```python
from build123d import *

# Parameters (mm, degrees)
SKETCH1_R           = 141.81
SKETCH1_R_2         = 119.99
BOSS_EXTRUDE1_DEPTH = 10.91
CUT_EXTRUDE1_START  = -10.91
SKETCH2_W           = 21.82
SKETCH2_H           = 10.91
SKETCH2_W_2         = 10.91
SKETCH2_H_2         = 21.82
CUT_EXTRUDE1_DEPTH  = 10.91
SKETCH3_R           = 5.455
CUT_EXTRUDE2_DEPTH  = 10.91


with BuildPart() as part:
    # Sketch1 → Boss-Extrude1 (new body)
    with BuildSketch(Plane(origin=(0, 0, 0), x_dir=(1, 0, 0), z_dir=(0, 1, 0))):
        with Locations(Location((0, 0, 0), (0, 0, 270))):
            Circle(SKETCH1_R)
        with Locations(Location((0, 0, 0), (0, 0, 270))):
            Circle(SKETCH1_R_2, mode=Mode.SUBTRACT)
    extrude(amount=BOSS_EXTRUDE1_DEPTH)

    # Sketch2 → Cut-Extrude1 (cut)
    with BuildSketch(Plane(origin=(0, 10.91, 0), x_dir=(1, 0, 0), z_dir=(0, 1, 0)).offset(CUT_EXTRUDE1_START)):
        with BuildLine():
            Line((-5.455, -130.9), (-5.455, -141.705042518))
            ThreePointArc((-5.455, -141.705042518), (0, -141.81), (5.455, -141.705042518))
            Line((5.455, -141.705042518), (5.455, -130.9))
            Line((5.455, -130.9), (0, -130.9))
            Line((0, -130.9), (-5.455, -130.9))
        make_face()
        Polygon((-71.635831422, -134.986899666), (-60.725831422, -116.090225355), (-70.174168578, -110.635225355), (-81.084168578, -129.531899666), align=None)
        Polygon((-129.531899666, -81.084168578), (-110.635225355, -70.174168578), (-116.090225355, -60.725831422), (-134.986899666, -71.635831422), align=None)
        with Locations((-141.81, 0)):
            Rectangle(SKETCH2_W, SKETCH2_H)
        Polygon((-134.986899666, 71.635831422), (-116.090225355, 60.725831422), (-110.635225355, 70.174168578), (-129.531899666, 81.084168578), align=None)
        Polygon((-81.084168578, 129.531899666), (-70.174168578, 110.635225355), (-60.725831422, 116.090225355), (-71.635831422, 134.986899666), align=None)
        with Locations((0, 141.81)):
            Rectangle(SKETCH2_W_2, SKETCH2_H_2)
        Polygon((71.635831422, 134.986899666), (60.725831422, 116.090225355), (70.174168578, 110.635225355), (81.084168578, 129.531899666), align=None)
        Polygon((129.531899666, 81.084168578), (110.635225355, 70.174168578), (116.090225355, 60.725831422), (134.986899666, 71.635831422), align=None)
        with Locations((141.81, 0)):
            Rectangle(SKETCH2_W, SKETCH2_H)
        Polygon((134.986899666, -71.635831422), (116.090225355, -60.725831422), (110.635225355, -70.174168578), (129.531899666, -81.084168578), align=None)
        Polygon((81.084168578, -129.531899666), (70.174168578, -110.635225355), (60.725831422, -116.090225355), (71.635831422, -134.986899666), align=None)
    extrude(amount=CUT_EXTRUDE1_DEPTH, mode=Mode.SUBTRACT)

    # Sketch3 → Cut-Extrude2 (cut)
    with BuildSketch(Plane(origin=(0, 10.91, 0), x_dir=(1, 0, 0), z_dir=(0, 1, 0))):
        with Locations(Location((-33.646658285, -125.571038224, 0), (0, 0, 270))):
            Circle(SKETCH3_R)
        with Locations(Location((-91.924379939, -91.924379939, 0), (0, 0, 270))):
            Circle(SKETCH3_R)
        with Locations(Location((-125.571038224, -33.646658285, 0), (0, 0, 270))):
            Circle(SKETCH3_R)
        with Locations(Location((-125.571038224, 33.646658285, 0), (0, 0, 270))):
            Circle(SKETCH3_R)
        with Locations(Location((-91.924379939, 91.924379939, 0), (0, 0, 270))):
            Circle(SKETCH3_R)
        with Locations(Location((-33.646658285, 125.571038224, 0), (0, 0, 270))):
            Circle(SKETCH3_R)
        with Locations(Location((33.646658285, 125.571038224, 0), (0, 0, 270))):
            Circle(SKETCH3_R)
        with Locations(Location((91.924379939, 91.924379939, 0), (0, 0, 270))):
            Circle(SKETCH3_R)
        with Locations(Location((125.571038224, 33.646658285, 0), (0, 0, 270))):
            Circle(SKETCH3_R)
        with Locations(Location((125.571038224, -33.646658285, 0), (0, 0, 270))):
            Circle(SKETCH3_R)
        with Locations(Location((91.924379939, -91.924379939, 0), (0, 0, 270))):
            Circle(SKETCH3_R)
        with Locations(Location((33.646658285, -125.571038224, 0), (0, 0, 270))):
            Circle(SKETCH3_R)
    extrude(amount=-CUT_EXTRUDE2_DEPTH, mode=Mode.SUBTRACT)


solid = part.part
```
Source: CAD feature listing. Evaluate the final solid. Frame: model axes, mm. A direction names the side the tool comes from. Round coordinates to 2 decimals unless told otherwise and drop trailing zeros. Write each loop counter-clockwise with the first axis right and the second up, starting at its lowest first coordinate (ties: lowest second). Pieces come first, ordered by that corner, then holes. Notation, with made-up numbers: M -14,53 L -1,53 A26 ccw -1,69 Z; hole C -7.5,-33.75 d1. An arc over 180 degrees is marked long. Use CSV: the item, a comma, the result in double quotes. Start each with the question number.
Q1. Cut plane B-B on x = 0. Output: boundary loops of the cut face in (y, z).
Q2. Pull-direction query (Z, two-part tool) for faces 6 (the face through (-36.275, 5.379, -137.092)), 7 (the face through (-65.384, 5.379, 113.401)), 8 (the face through (-5.455, 5, -136)), 9 (the face through (65.516, 5.379, 113.325)); classes: +Z half, -Z half, draft (parallel to the pull), parting line (faces both ways), or undercut.
Q3. Line query: line 1 (X direction, y = 6.5, z = -2.5); line 2 (X direction, y = 8.5, z = 61); line 3 (X direction, y = 5, z = 66). Output: solid intervals per line, ascending. Write a range as from..to.
Q4. Access query for faces 1 (the face through (0, 5, 130.9)), 2 (the face through (136, 5, -5.455)), 3 (the face through (72.84, 5.38, -115.25)), 4 (the face through (-137.092, 5.379, 36.275)), 5 (the face through (63.389, 5.379, 120.703)). Directions: +Z, -Z, +X, -X, +Y, -Y. A direction counts if a zero-diameter tool reaches every point of the face in a straight line with its end or side. Return the directions, or none.
Q5. Cut plane C-C on y = 3.5. Count the separate pieces of the cut face and the enclosed holes in it, plus the area to 3 significant figures.
Q6. First-contact query: P1, Ø1, axis at y = 2, z = 82.5, coming from the -X side; P2, Ø1.5, axis at x = -59.5, y = 2.5, coming from the +Z side; P3, Ø14, axis at x = 125.57, z = -33.65, coming from the -Y side; P4, Ø5.5, axis at x = 1.5, y = 4.5, coming from the -Z side. Flat tips, straight axial feed; report the tip coordinate or a pass-through.
Q7. Cut plane A-A on z = 0. Output: boundary loops of the cut face in (x, y).
Results found:
1,outline,"M 0,-130.9 L 10.91,-130.9 L 10.91,-119.99 L 0,-119.99 Z; M 0,119.99 L 10.91,119.99 L 10.91,130.9 L 0,130.9 Z"
2,face 6,"-Z half"
2,face 7,"undercut"
2,face 8,"draft"
2,face 9,"undercut"
3,line 1,"-130.9..-119.96, 119.96..130.9"
3,line 2,"-128.02..-116.57, -115.93..-103.33, 103.33..115.93, 116.57..128.02"
3,line 3,"-125.52..-125.23, -113.05..-100.21, 100.21..113.05, 125.23..125.52"
4,face 1,"+Z, +Y, -Y"
4,face 2,"+X, +Y, -Y"
4,face 3,"-Z, +Y, -Y"
4,face 4,"+Z, -X, +Y, -Y"
4,face 5,"+Y, -Y"
5,separate pieces,"1"
5,enclosed holes,"13"
5,area,"15,400 mm^2"
6,P1,"x = -115.7"
6,P2,"z = 129.07"
6,P3,"y = 0"
6,P4,"z = -130.9"
7,outline,"M -130.9,0 L -119.99,0 L -119.99,10.91 L -130.9,10.91 Z; M 119.99,0 L 130.9,0 L 130.9,10.91 L 119.99,10.91 Z"
